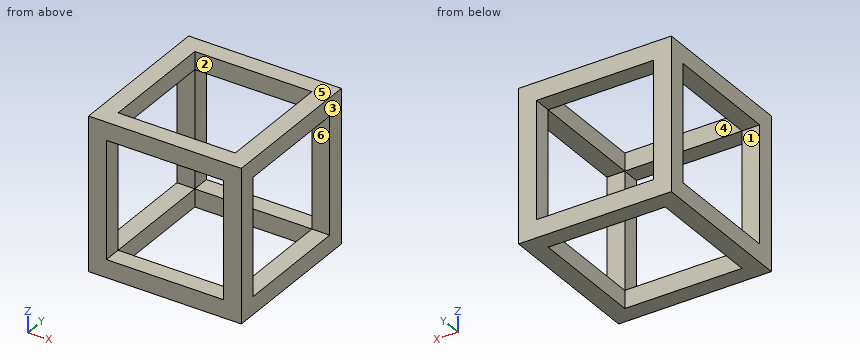
from build123d import *

# Parameters (mm, degrees)
F0_W     = 30
F0_H     = 30
F1_DEPTH = 30
F2_W     = 23
F2_H     = 23
F3_DEPTH = 30
F4_W     = 23
F4_H     = 23
F5_DEPTH = 30
F6_W     = 23
F6_H     = 23
F7_DEPTH = 30


with BuildPart() as f1:
    # F0 (on Front) → F1 (new body)
    with BuildSketch(Plane.XZ):
        Rectangle(F0_W, F0_H)
    extrude(amount=F1_DEPTH)

    # F2 (on face) → F3 (cut)
    with BuildSketch(Plane(origin=(0, 0, 0), x_dir=(-1, 0, 0), z_dir=(0, 1, 0))):
        Rectangle(F2_W, F2_H)
    extrude(amount=-F3_DEPTH, mode=Mode.SUBTRACT)

    # F4 (on face) → F5 (cut)
    with BuildSketch(Plane(origin=(-15, 0, 0), x_dir=(0, -1, 0), z_dir=(-1, 0, 0))):
        with Locations((15, 0)):
            Rectangle(F4_W, F4_H)
    extrude(amount=-F5_DEPTH, mode=Mode.SUBTRACT)

    # F6 (on face) → F7 (cut)
    with BuildSketch(Plane.XY.offset(15)):
        with Locations((0, -15)):
            Rectangle(F6_W, F6_H)
    extrude(amount=-F7_DEPTH, mode=Mode.SUBTRACT)


solid = f1.part
Check sheet for the modelled part. Datum: model origin and axes. Units: mm. Face numbers are marked on the shaded views. A direction names the side the tool comes from. Round coordinates to 2 decimals unless told otherwise and drop trailing zeros. Loops run counter-clockwise (first coordinate to the right, second up) from the corner with the lowest first, then second, coordinate; pieces in that order, holes last. Notation, with made-up numbers: (33.25, 73) - (51.25, 73) arc R23 cw to (51.25, 96) - close; hole circle Ø2 at (81.5, 12.25). An arc over 180 degrees is marked (long way). Answer as CSV lines item,"result". Start each with the question number.
Item 1: Release check for a two-part mould opening along X. For the marked faces 1, 2 and 3 record: +X half, -X half, draft (parallel to the pull), parting line (faces both ways), or undercut.
Item 2: Scan lines: line 1 (Z direction, x = 6.5, y = -27); line 2 (Y direction, x = 13.25, z = -9.75). Record each from-to range of solid material in increasing order. Write a range as [from, to].
Item 3: Section check A-A (y = -21). Record the boundary of the cut face in (x, z).
Item 4: Depth check by flat-ended pin: P1, Ø3, axis at x = 14, z = -5, coming from the +Y side; P2, Ø8, axis at x = -5, z = -0.5, coming from the -Y side. Enter the tip coordinate at first touch or a pass-through.
Item 5: Section check D-D (x = -12.5). Record the boundary of the cut face in (y, z).
Item 6: Section check B-B (x = 3.5). Record the boundary of the cut face in (y, z), and give its area (3 significant figures).
Item 7: Section check C-C (y = -27.5). Record the boundary of the cut face in (x, z), and give its area (3 significant figures).
Item 8: Set-up check for the marked faces 4, 5 and 6: record each of +Z, -Z, +X, -X, +Y, -Y from which the full face is reachable in a straight line by a thin tool's end or side.
Report:
1,face 1,"draft"
1,face 2,"undercut"
1,face 3,"+X half"
2,line 1,"z = [-15, -11.5], [11.5, 15]"
2,line 2,"y = [-30, -26.5], [-3.5, 0]"
3,outline,"(-15, -15) - (-11.5, -15) - (-11.5, -11.5) - (-15, -11.5) - close; (-15, 11.5) - (-11.5, 11.5) - (-11.5, 15) - (-15, 15) - close; (11.5, -15) - (15, -15) - (15, -11.5) - (11.5, -11.5) - close; (11.5, 11.5) - (15, 11.5) - (15, 15) - (11.5, 15) - close"
4,P1,"stops at y = 0"
4,P2,"passes through"
5,outline,"(-30, -15) - (0, -15) - (0, 15) - (-30, 15) - close; hole (-26.5, -11.5) - (-3.5, -11.5) - (-3.5, 11.5) - (-26.5, 11.5) - close"
6,outline,"(-30, -15) - (-26.5, -15) - (-26.5, -11.5) - (-30, -11.5) - close; (-30, 11.5) - (-26.5, 11.5) - (-26.5, 15) - (-30, 15) - close; (-3.5, -15) - (0, -15) - (0, -11.5) - (-3.5, -11.5) - close; (-3.5, 11.5) - (0, 11.5) - (0, 15) - (-3.5, 15) - close"
6,area,"49.0 mm2"
7,outline,"(-15, -15) - (15, -15) - (15, 15) - (-15, 15) - close; hole (-11.5, -11.5) - (11.5, -11.5) - (11.5, 11.5) - (-11.5, 11.5) - close"
7,area,"371 mm2"
8,face 4,"+Z, -Z"
8,face 5,"+Z, +X, -X, +Y, -Y"
8,face 6,"+X, -X"
